Part model, mm, in its own coordinate system. A direction names the side the tool comes from. Coordinates: 2 decimals unless noted, no trailing zeros. Order: outer loops, then holes, each group sorted by start corner. A loop starts at its lowest first (then second) coordinate and runs counter-clockwise, first axis right, second up.
1) Cut at B-B (z = -23). List the corners of the cut face in (x, y), and give its area (3 significant figures).
2) Cut at C-C (z = -57.5). List the corners of the cut face in (x, y) (3 decimals), and give its area (3 significant figures).
3) Wall check: L1, parallel to X at y = 9, z = -57.5 (3 decimals); L2, parallel to Z at x = -78.45, y = 7.5 (3 decimals); L3, parallel to Y at x = 5, z = 5. Give the ranges that are in metal, low to high.
4) Pin check, flat tips, straight feed: pin 1 Ø3.5 at (y, z) = (8, -4.5) entering from +X; pin 2 Ø4 at (x, y) = (-40.5, 4) entering from +Z; pin 3 Ø8 at (x, z) = (-23.5, 20.5) entering from +Y. Stop position of each tip, or through.
5) Tool access for faces 1 (the cylindrical face through (-82.83, 9.06, -59.91)), 2 (the flat face through (50.89, 2.46, 31.1)), 3 (the flat face through (11, 8, 11.736)), 4 (the flat face through (-15.385, 8, 0)), 5 (the flat face through (-50.006, 2.465, 30.444)): list every direction of +Z, -Z, +X, -X, +Y, -Y with a clear straight run to the whole face (end or side of a thin tool).
6) Cut at A-A (x = 34). List the corners of the cut face in (y, z).
7) Cut at D-D (x = -78.45). List the corners of the cut face in (y, z) (3 decimals).
8) Mould opens along Y. For faces 6 (the cylindrical face through (-79.47, 7.4, -58.83)), 7 (the flat face through (79, 15, -55)), 8 (the flat face through (7.514, 7, 0)) say: +Y half, -Y half, draft (parallel to the pull), parting line (faces both ways), or undercut.
```python
from build123d import *

# Parameters (mm, degrees)
SKETCH2_R           = 1.675
BOSS_EXTRUDE2_DEPTH = 5
SKETCH4_R           = 5
SKETCH4_R_2         = 1.675
BOSS_EXTRUDE3_DEPTH = 10
SKETCH7_W           = 7.89896268
SKETCH7_H           = 23.466499487
BOSS_EXTRUDE4_DEPTH = 4
BOSS_EXTRUDE5_DEPTH = 3


with BuildPart() as part:
    # Sketch2 → Boss-Extrude2 (new body)
    with BuildSketch(Plane(origin=(0, 0, 0), x_dir=(1, 0, 0), z_dir=(0, 1, 0))):
        with BuildLine():
            Line((-5.927337077, 10.543675079), (-75.494184373, 61.532760094))
            ThreePointArc((-75.494184373, 61.532760094), (-82.4827602, 60.455815483), (-81.405815339, 53.467239694))
            Line((-81.405815339, 53.467239694), (-19.473220794, 8.073687288))
            ThreePointArc((-19.473220794, 8.073687288), (-15.384851579, 0.009024421), (-19.471837334, -8.056339641))
            Line((-19.471837334, -8.056339641), (-81.406507067, -53.467746788))
            ThreePointArc((-81.406507067, -53.467746788), (-82.482253212, -60.456507067), (-75.493492933, -61.532253212))
            Line((-75.493492933, -61.532253212), (-5.946235564, -10.53918529))
            ThreePointArc((-5.946235564, -10.53918529), (-0.035497695, -8.603691918), (5.87612073, -10.53649412))
            Line((5.87612073, -10.53649412), (75.495328977, -61.533598783))
            ThreePointArc((75.495328977, -61.533598783), (82.483179585, -60.455243211), (81.405815339, -53.467239694))
            Line((81.405815339, -53.467239694), (19.501443033, -8.094372803))
            ThreePointArc((19.501443033, -8.094372803), (15.413073818, -0.029709936), (19.500059572, 8.035654125))
            Line((19.500059572, 8.035654125), (81.426238752, 53.440835874))
            ThreePointArc((81.426238752, 53.440835874), (82.509164133, 60.476238742), (75.473761267, 61.55916414))
            Line((75.473761267, 61.55916414), (5.897307879, 10.54468927))
            ThreePointArc((5.897307879, 10.54468927), (-0.014848637, 8.609195675), (-5.927337077, 10.543675079))
        make_face()
        with Locations(Location((-78.45, 57.5, 0), (0, 0, 270))):
            Circle(SKETCH2_R, mode=Mode.SUBTRACT)
        with Locations(Location((-78.45, -57.5, 0), (0, 0, 270))):
            Circle(SKETCH2_R, mode=Mode.SUBTRACT)
        with Locations(Location((78.45, 57.5, 0), (0, 0, 270))):
            Circle(SKETCH2_R, mode=Mode.SUBTRACT)
        with Locations(Location((78.45, -57.5, 0), (0, 0, 270))):
            Circle(SKETCH2_R, mode=Mode.SUBTRACT)
    extrude(amount=BOSS_EXTRUDE2_DEPTH)

    # Sketch4 → Boss-Extrude3 (add)
    # profile 1 of 4: a face of its own
    with BuildSketch(Plane(origin=(0, 5, 0), x_dir=(1, 0, 0), z_dir=(0, 1, 0))):
        with Locations(Location((-78.45, 57.5, 0), (0, 0, 53.760412974))):
            Circle(SKETCH4_R)
        with Locations(Location((-78.45, 57.5, 0), (0, 0, 270))):
            Circle(SKETCH4_R_2, mode=Mode.SUBTRACT)
    # profile 2 of 4: a face of its own
    with BuildSketch(Plane(origin=(0, 5, 0), x_dir=(1, 0, 0), z_dir=(0, 1, 0))):
        with Locations(Location((78.45, 57.5, 0), (0, 0, 270))):
            Circle(SKETCH4_R)
        with Locations(Location((78.45, 57.5, 0), (0, 0, 270))):
            Circle(SKETCH4_R_2, mode=Mode.SUBTRACT)
    # profile 3 of 4: a face of its own
    with BuildSketch(Plane(origin=(0, 5, 0), x_dir=(1, 0, 0), z_dir=(0, 1, 0))):
        with Locations(Location((-78.45, -57.5, 0), (0, 0, 126.24941546))):
            Circle(SKETCH4_R)
        with Locations(Location((-78.45, -57.5, 0), (0, 0, 270))):
            Circle(SKETCH4_R_2, mode=Mode.SUBTRACT)
    # profile 4 of 4: a face of its own
    with BuildSketch(Plane(origin=(0, 5, 0), x_dir=(1, 0, 0), z_dir=(0, 1, 0))):
        with Locations(Location((78.45, -57.5, 0), (0, 0, 53.760412974))):
            Circle(SKETCH4_R)
        with Locations(Location((78.45, -57.5, 0), (0, 0, 270))):
            Circle(SKETCH4_R_2, mode=Mode.SUBTRACT)
    extrude(amount=BOSS_EXTRUDE3_DEPTH)

    # Sketch7 → Boss-Extrude4 (add)
    with BuildSketch(Plane(origin=(0, 5, 0), x_dir=(1, 0, 0), z_dir=(0, 1, 0))):
        Polygon((-15.384851579, 0.009024421), (-15.384851579, -11.66808167), (-7.485888899, -11.66808167), (-7.485888899, -0.137260517), (-7.485888899, 11.686017077), (-15.384851579, 11.686017077), align=None)
        with Locations((11.463592441, -0.003096667)):
            Rectangle(SKETCH7_W, SKETCH7_H)
    extrude(amount=BOSS_EXTRUDE4_DEPTH)

    # Sketch8 → Boss-Extrude5 (add)
    with BuildSketch(Plane(origin=(0, 9, 0), x_dir=(1, 0, 0), z_dir=(0, 1, 0))):
        with BuildLine():
            Line((-15.384851579, -11.722899791), (-7.485888899, -11.66808167))
            Line((-7.485888899, -11.66808167), (-5.943452184, -10.53498393))
            ThreePointArc((-5.943452184, -10.53498393), (0.004475009, -8.594141897), (5.941608561, -10.567755551))
            Line((5.941608561, -10.567755551), (7.514111101, -11.73634641))
            Line((7.514111101, -11.73634641), (15.413073781, -11.73634641))
            Line((15.413073781, -11.73634641), (15.413073781, 11.730153077))
            Line((15.413073781, 11.730153077), (7.514111101, 11.730153077))
            Line((7.514111101, 11.730153077), (5.94895034, 10.569274798))
            ThreePointArc((5.94895034, 10.569274798), (0.014632257, 8.601189918), (-5.928647633, 10.542043685))
            Line((-5.928647633, 10.542043685), (-7.485888899, 11.686017077))
            Line((-7.485888899, 11.686017077), (-15.384851579, 11.686017077))
            Line((-15.384851579, 11.686017077), (-15.384851579, -11.722899791))
        make_face()
    extrude(amount=BOSS_EXTRUDE5_DEPTH)


solid = part.part
```
Geometry check:
1. outline: (-39.84, 0) - (-22.92, 0) - (-22.92, 5) - (-39.84, 5) - close; (22.88, 0) - (39.91, 0) - (39.91, 5) - (22.88, 5) - close
1. area: 170 mm2
2. outline: (-83.45, 0) - (-80.125, 0) - (-80.125, 15) - (-83.45, 15) - close; (-76.775, 0) - (-69.992, 0) - (-69.992, 5) - (-73.45, 5) - (-73.45, 15) - (-76.775, 15) - close; (69.938, 0) - (76.775, 0) - (76.775, 15) - (73.45, 15) - (73.45, 5) - (69.938, 5) - close; (80.125, 0) - (83.483, 0) - (83.483, 5) - (83.45, 5) - (83.45, 15) - (80.125, 15) - close
2. area: 235 mm2
3. L1: x = -83.45 to -80.125, -76.775 to -73.45, 73.45 to 76.775, 80.125 to 83.45
3. L2: z = -62.5 to -59.175, -55.825 to -52.5, 52.5 to 55.825, 59.175 to 62.5
3. L3: y = 0 to 5, 9 to 12
4. pin 1: stops at x = 15.41
4. pin 2: stops at z = 37.34
4. pin 3: stops at y = 5
5. face 1: +Y
5. face 2: +X, +Y, -Y
5. face 3: +Z, +X, -X, +Y
5. face 4: +Z, -Z, -X, +Y
5. face 5: -X, +Y, -Y
6. outline: (0, -31.15) - (5, -31.15) - (5, -18.67) - (0, -18.67) - close; (0, 18.72) - (5, 18.72) - (5, 31.14) - (0, 31.14) - close
7. outline: (0, -62.5) - (15, -62.5) - (15, -59.175) - (0, -59.175) - close; (0, -55.825) - (15, -55.825) - (15, -52.5) - (5, -52.5) - (5, -51.301) - (0, -51.301) - close; (0, 51.3) - (5, 51.3) - (5, 52.5) - (15, 52.5) - (15, 55.825) - (0, 55.825) - close; (0, 59.175) - (15, 59.175) - (15, 62.5) - (0, 62.5) - close
8. face 6: draft
8. face 7: +Y half
8. face 8: undercut
